from build123d import *

# Parameters (mm, degrees)
ESTRUSIONE_ESTRUSIONE2_DEPTH  = 11
RACCORDO1_R                   = 3
SCHIZZO2_R                    = 4
TAGLIO_ESTRUSIONE1_DEPTH      = 16
SCHIZZO2_3_R                  = 6
SCHIZZO2_3_R_2                = 4
TAGLIO_ESTRUSIONE2_DEPTH      = 4
RACCORDO2_R                   = 1
SCHIZZO3_W                    = 40.5
SCHIZZO3_H                    = 8
TAGLIO_ESTRUSIONE4_DEPTH      = 46
TAGLIO_ESTRUSIONE4_DEPTH_BACK = 1
SCHIZZO4_R                    = 4
TAGLIO_ESTRUSIONE5_DEPTH      = 23
SMUSSO1_SIZE                  = 1


with BuildPart() as part:
    # Schizzo1 → Estrusione-Estrusione2 (new body, symmetric)
    with BuildSketch(Plane.XY):
        with BuildLine():
            Line((0, 0), (0, 15))
            Line((0, 15), (25, 15))
            Line((25, 15), (43.5, 19.95706006))
            Line((43.5, 19.95706006), (43.5, 37.5))
            Line((43.5, 37.5), (41, 37.5))
            Line((41, 37.5), (41, 45))
            Line((41, 45), (51.395196715, 45))
            Line((51.395196715, 45), (60.912678196, 15.708203932))
            ThreePointArc((60.912678196, 15.708203932), (59.208203932, 4.946576972), (49.5, 0))
            Line((49.5, 0), (0, 0))
        make_face()
    extrude(amount=ESTRUSIONE_ESTRUSIONE2_DEPTH, both=True)

    # Raccordo1
    raccordo1_edges = [part.edges().sort_by_distance(p)[0] for p in [
        (51.395196715, 45, 0),
    ]]
    fillet(raccordo1_edges, radius=RACCORDO1_R)

    # Schizzo2 → Taglio-Estrusione1 (cut, through all)
    with BuildSketch(Plane(origin=(0, 15, 0), x_dir=(1, 0, 0), z_dir=(0, 1, 0))):
        with Locations((10, 0)):
            Circle(SCHIZZO2_R)
    extrude(amount=-TAGLIO_ESTRUSIONE1_DEPTH, mode=Mode.SUBTRACT)

    # Schizzo2<3> → Taglio-Estrusione2 (cut)
    with BuildSketch(Plane(origin=(0, 15, 0), x_dir=(1, 0, 0), z_dir=(0, 1, 0))):
        with Locations((10, 0)):
            Circle(SCHIZZO2_3_R)
        with Locations((10, 0)):
            Circle(SCHIZZO2_3_R_2, mode=Mode.SUBTRACT)
    extrude(amount=-TAGLIO_ESTRUSIONE2_DEPTH, mode=Mode.SUBTRACT)

    # Raccordo2
    raccordo2_edges = [part.edges().sort_by_distance(p)[0] for p in [
        (41, 37.5, 0),
        (41, 45, 0),
    ]]
    fillet(raccordo2_edges, radius=RACCORDO2_R)

    # Schizzo3 → Taglio-Estrusione4 (cut, two sides)
    with BuildSketch(Plane(origin=(0, 0, 0), x_dir=(1, 0, 0), z_dir=(0, 1, 0))) as taglio_estrusione4_sk:
        with Locations((41.25, 0)):
            Rectangle(SCHIZZO3_W, SCHIZZO3_H)
    extrude(amount=TAGLIO_ESTRUSIONE4_DEPTH, mode=Mode.SUBTRACT)
    extrude(taglio_estrusione4_sk.sketch, amount=-TAGLIO_ESTRUSIONE4_DEPTH_BACK, mode=Mode.SUBTRACT)

    # Schizzo4 → Taglio-Estrusione5 (cut, through all)
    with BuildSketch(Plane.XY.offset(11)):
        with Locations((32, 7.5)):
            Circle(SCHIZZO4_R)
    extrude(amount=-TAGLIO_ESTRUSIONE5_DEPTH, mode=Mode.SUBTRACT)

    # Smusso1
    smusso1_edges = [part.edges().sort_by_distance(p)[0] for p in [
        (28, 7.5, -11),
        (28, 7.5, 11),
    ]]
    chamfer(smusso1_edges, length=SMUSSO1_SIZE)


solid = part.part
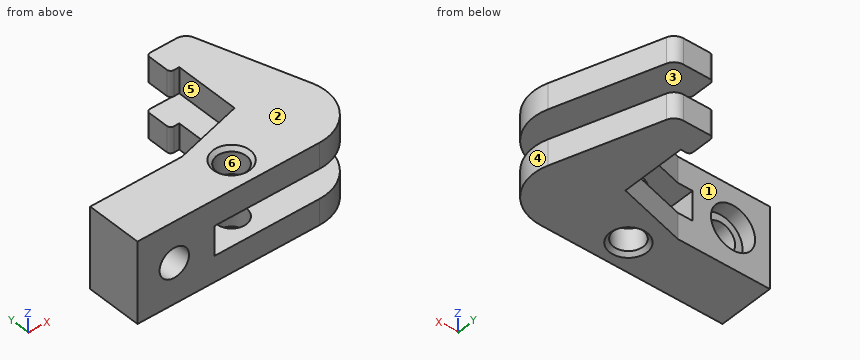
Source: CAD feature listing. Evaluate the final solid. Frame: model axes, mm. Face numbers are marked on the shaded views. A direction names the side the tool comes from. Coordinates: 2 decimals unless noted, no trailing zeros. Order: outer loops, then holes, each group sorted by start corner. A loop starts at its lowest first (then second) coordinate and runs counter-clockwise, first axis right, second up.
Item 1: Cut plane C-C (x = 10). Return loops of the section in (y, z).
Output values:
outline: (0, -11) - (15, -11) - (15, -6) - (11, -6) - (11, -4) - (0, -4) - close; (0, 4) - (11, 4) - (11, 6) - (15, 6) - (15, 11) - (0, 11) - close
Item 2: Cut plane A-A (z = 0). Return loops of the section in (x, y), plus the area to 3 significant figures.
Output values:
outline: (0, 0) - (6, 0) - (6, 11) - (4, 11) - (4, 15) - (0, 15) - close; (14, 0) - (21, 0) - (21, 15) - (16, 15) - (16, 11) - (14, 11) - close
area: 179 mm2
Item 3: Pull-direction query (X, two-part tool) for the marked faces 4, 5 and 6; classes: pulls with the +X half, pulls with the -X half, needs draft (parallel to the pull), parting line crosses it, or undercut.
Output values:
face 4: pulls with the +X half
face 5: pulls with the -X half
face 6: undercut
Item 4: Material intervals for line 1 (Z direction, x = 10, y = 13.85); line 2 (Z direction, x = 10, y = 6); line 3 (X direction, y = 2.5, z = 0), sorted ascending.
Output values:
line 1: z = -11 to -6, 6 to 11
line 2: z = -11 to -4, 4 to 11
line 3: x = 0 to 6, 14 to 21
Item 5: Cut plane D-D (y = 41.5). Return loops of the section in (x, z), plus the area to 3 significant figures.
Output values:
outline: (41, -11) - (52.53, -11) - (52.53, -4) - (41, -4) - close; (41, 4) - (52.53, 4) - (52.53, 11) - (41, 11) - close
area: 161 mm2
Item 6: First-contact query: P1, Ø10, axis at x = 9, z = -4.5, coming from the +Y side; P2, Ø9, axis at x = 32, y = 7.5, coming from the -Z side; P3, Ø2, axis at y = 26.5, z = 7, coming from the -X side. Flat tips, straight axial feed; report the tip coordinate or a pass-through.
Output values:
P1: stops at y = 15
P2: stops at z = -10.5
P3: stops at x = 43.5
Item 7: Set-up query: the marked faces 1, 2 and 3. Return all of +Z, -Z, +X, -X, +Y, -Y with unobstructed straight access to the full face (end or side cutting, diameter ignored); none if empty.
Output values:
face 1: +Z, -Z, -X, +Y
face 2: +Z, +X, -X, +Y, -Y
face 3: +X, +Y, -Y
Item 8: Cut plane B-B (y = 7.5). Return loops of the section in (x, z).
Output values:
outline: (0, -11) - (27, -11) - (28, -10) - (28, -4) - (21, -4) - (21, 4) - (28, 4) - (28, 10) - (27, 11) - (0, 11) - close; (36, -10) - (37, -11) - (60.62, -11) - (60.62, -4) - (36, -4) - close; (36, 4) - (60.62, 4) - (60.62, 11) - (37, 11) - (36, 10) - close; hole circle Ø8 at (10, 0)
